Autodesk Inventor part; units mm, degrees
ref_plane "YZ Plane" through (0, 0, 0) normal (1, 0, 0) x (0, 1, 0)
ref_plane "XZ Plane" through (0, 0, 0) normal (0, 1, 0) x (-1, 0, 0)
ref_plane "XY Plane" through (0, 0, 0) normal (0, 0, 1) x (1, 0, 0)
sketch "Sketch1" plane through (0, 0, 0) normal (0, 1, 0) x (-1, 0, 0)
  line L0 (77.5, 40) -> (-77.5, 40)
  line L1 (-77.5, 40) -> (-77.5, -40)
  line L2 (-77.5, -40) -> (77.5, -40)
  line L3 (77.5, -40) -> (77.5, 40)
  point P0 (0, 0)
  point P1 (0, -40)
  point P2 (77.5, 0)
  dimension "d0" = 155
  dimension "d1" = 80
extrude "Extrusion1" add sketch "Sketch1" along normal blind 1
sketch "Sketch3" plane through (0, 1, 0) normal (0, 1, 0) x (1, 0, 0)
  line L0 (77.5, 40) -> (-77.5, 40)
  line L1 (-77.5, -40) -> (77.5, -40)
  line L2 (-68.3973, 40) -> (61.6027, 40)
  line L3 (61.6027, 40) -> (61.6027, -40)
  line L4 (61.6027, -40) -> (-68.3973, -40)
  line L5 (-68.3973, -40) -> (-68.3973, 40)
  point P0 (0, 0)
  point P1 (0, 40)
  dimension "d7" = 130
extrude "Extrusion2" add sketch "Sketch3" along normal blind 40
properties part number "sound amplifier"
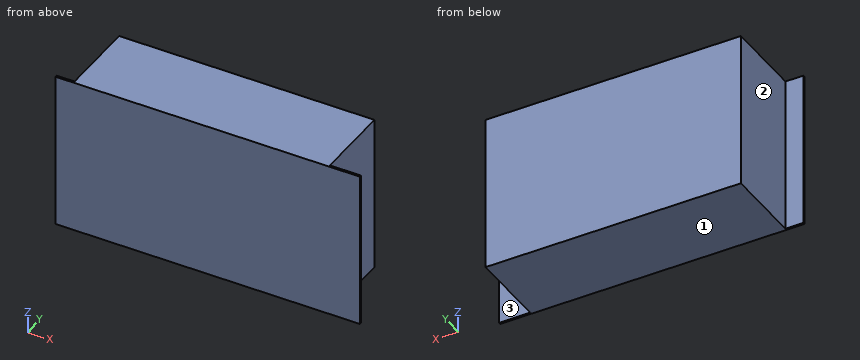
Read the model definition and answer for the solid it produces. Units are mm, in the model's axes. Face numbers are marked on the shaded views. A direction names the side the tool comes from. Give positions to 0.01 mm unless a question says otherwise; leave off trailing zeros. Write each loop counter-clockwise with the first axis right and the second up, starting at its lowest first coordinate (ties: lowest second). Pieces come first, ordered by that corner, then holes. Notation, with made-up numbers: M -34,23.5 L -22,23.5 A14 cw -22,48.5 Z; hole C 68,70 d1. An arc over 180 degrees is marked long. Put each result on its own line as item: value. Start each with the question number.
1. The part is cut by section A-A, the plane z = 11.5. Give the vertices of the cut face in (x, y).
2. The part is cut by section B-B, the plane x = 65.5. Give the vertices of the cut face in (y, z).
3. Which of the six approach directions +Z, -Z, +X, -X, +Y, -Y give full straight-line access (tool end or side, diameter ignored) to the marked faces 1, 2 and 3?
4. The part is cut by section C-C, the plane y = 20. Give the vertices of the cut face in (x, z).
5. Consider line 1 along X through (y, z) = (37.5, 17); line 2 along Y through (x, z) = (65.5, 34). Determine where each line is inside the solid, lowest interval first.
6. Each of these flat-tipped pins is pushed along its axis until it touches: pin 1 Ø8 at (x, z) = (66.5, -8.5) entering from +Y; pin 2 Ø10 at (y, z) = (34, 18) entering from +X; pin 3 Ø10 at (y, z) = (28.5, -5) entering from -X. Where does it stop, or does it pass through?
Final values:
1. outline: M -77.5,0 L 77.5,0 L 77.5,1 L 61.6,1 L 61.6,41 L -68.4,41 L -68.4,1 L -77.5,1 Z
2. outline: M 0,-40 L 1,-40 L 1,40 L 0,40 Z
3. face 1: -Z, +X, -X, +Y, -Y
3. face 2: +Z, -Z, -X, +Y
3. face 3: +Z, -Z, +X, +Y
4. outline: M -68.4,-40 L 61.6,-40 L 61.6,40 L -68.4,40 Z
5. line 1: x = -68.4 to 61.6
5. line 2: y = 0 to 1
6. pin 1: stops at y = 1
6. pin 2: stops at x = 61.6
6. pin 3: stops at x = -68.4
